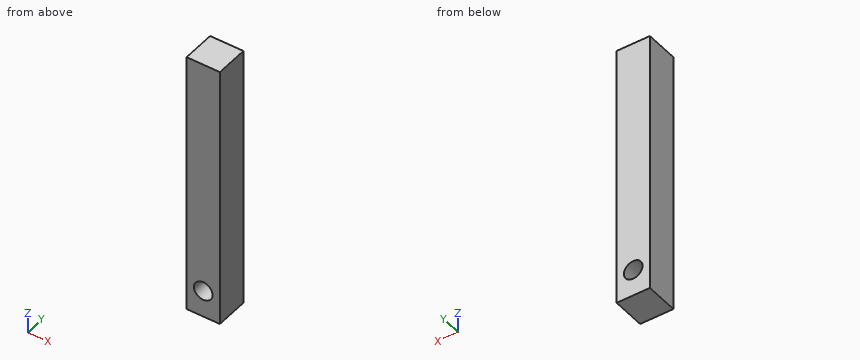
```python
from build123d import *

# Parameters (mm, degrees)
SKETCH_2_W          = 25.4
SKETCH_2_H          = 25.4
EXTRUDE_1_DEPTH     = 203.2
SKETCH_3_R          = 7.112
CUT_EXTRUDE_1_DEPTH = 207.350575478


with BuildPart() as part:
    # 草图2 → 凸台-拉伸1 (new body)
    with BuildSketch(Plane.XY):
        with Locations((12.7, 12.7)):
            Rectangle(SKETCH_2_W, SKETCH_2_H)
    extrude(amount=EXTRUDE_1_DEPTH)

    # 草图3 → 切除-拉伸1 (cut, through all)
    with BuildSketch(Plane(origin=(0, 25.4, 0), x_dir=(1, 0, 0), z_dir=(0, 1, 0))):
        with Locations(Location((12.7, -20.574, 0), (0, 0, 270))):
            Circle(SKETCH_3_R)
    extrude(amount=-CUT_EXTRUDE_1_DEPTH, mode=Mode.SUBTRACT)


solid = part.part
```
For this review, take the finished solid that the model builds, in its own axes (mm). Round coordinates to 2 decimals unless told otherwise and drop trailing zeros. Write each loop counter-clockwise with the first axis right and the second up, starting at its lowest first coordinate (ties: lowest second). Pieces come first, ordered by that corner, then holes. Notation, with made-up numbers: (34.5, 65.25) -> (86.5, 65.25) arc R35 cw to (86.5, 102.25) -> close; hole circle Ø3 at (82, 45.25). An arc over 180 degrees is marked (long way). Use one line per item in the form item = value.
1) Take a section at B-B, the plane y = 18.5. Write out the cut boundary in (x, z).
Found:
outline = (0, 0) -> (25.4, 0) -> (25.4, 203.2) -> (0, 203.2) -> close; hole circle Ø14.22 at (12.7, 20.57)
2) Take a section at A-A, the plane x = 12.7. Write out the cut boundary in (y, z), and give its area (3 significant figures).
Found:
outline = (0, 0) -> (25.4, 0) -> (25.4, 13.46) -> (0, 13.46) -> close; (0, 27.69) -> (25.4, 27.69) -> (25.4, 203.2) -> (0, 203.2) -> close
area = 4,800 mm2
3) To check wall thickness, follow L1, parallel to Z at x = 12.75, y = 1; L2, parallel to Z at x = 13.5, y = 9. State the ranges of each line that lie inside material, in increasing order. Write a range as from..to.
Found:
L1 = 0..13.46, 27.69..203.2
L2 = 0..13.51, 27.64..203.2
